Geometry: final body of the model. Coordinates: model frame, mm. Face numbers are marked on the shaded views. A direction names the side the tool comes from. Give positions to 0.01 mm unless a question says otherwise; leave off trailing zeros. Write each loop counter-clockwise with the first axis right and the second up, starting at its lowest first coordinate (ties: lowest second). Pieces come first, ordered by that corner, then holes.
Q1. Line query: line 1 (Z direction, x = -27, y = -7); line 2 (Y direction, x = 0, z = 3.65); line 3 (X direction, y = -13, z = -27.5). Output: solid intervals per line, ascending.
Q2. Pin query (flat end, axial travel): pin 1 Ø1 at (x, y) = (-5.5, 3.5) entering from -Z; pin 2 Ø3 at (y, z) = (19.5, -55.5) entering from +X; pin 3 Ø15 at (x, y) = (-15, 6) entering from +Z. Return the tip coordinate at first contact, or that it passes through.
Q3. Section A-A (z = -64). Return the cut outline in (x, y), plus the area to 3 significant figures.
Q4. Section D-D (x = -24). Return the cut outline in (y, z).
Q5. Section B-B (y = 13.5). Return the cut outline in (x, z).
Q6. Reachability of the marked faces 1 and 2 from +Z, -Z, +X, -X, +Y, -Y: full face, straight path, thin tool, end or side. Return the list, or none.
Q7. Section C-C (y = 0). Return the cut outline in (x, z).
Q8. Mould query, pull axis Z, two halves, no side actions, for the marked faces 3, 4 and 5. Classes: +Z half, -Z half, draft (parallel to the pull), parting line (faces both ways), or undercut.
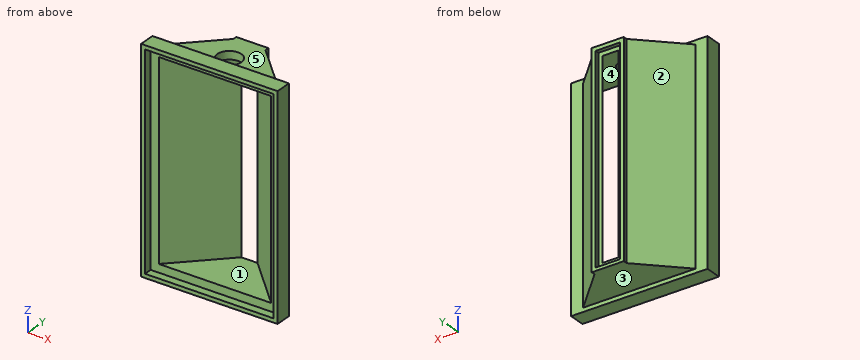
from build123d import *

# Parameters (mm, degrees)
SKETCH2_R            = 7.5
BOSS_EXTRUDE1_DEPTH  = 5
BOSS_EXTRUDE4_DEPTH  = 120
BOSS_EXTRUDE5_DEPTH  = 5
SKETCH7_W            = 85
SKETCH7_H            = 135
SKETCH7_W_2          = 70
SKETCH7_H_2          = 120
BOSS_EXTRUDE6_DEPTH  = 5
SKETCH10_W           = 85
SKETCH10_H           = 135
SKETCH10_W_2         = 80.1
SKETCH10_H_2         = 130.1
BOSS_EXTRUDE9_DEPTH  = 5
SKETCH11_W           = 20
SKETCH11_H           = 130
SKETCH11_W_2         = 15
SKETCH11_H_2         = 125.670447934
BOSS_EXTRUDE10_DEPTH = 2.5


with BuildPart() as part:
    # Sketch2 → Boss-Extrude1 (new body)
    with BuildSketch(Plane.XY):
        Polygon((-10, 17.5), (10, 17.5), (40, -12.5), (-40, -12.5), align=None)
        Circle(SKETCH2_R, mode=Mode.SUBTRACT)
    extrude(amount=BOSS_EXTRUDE1_DEPTH)

    # Sketch5 → Boss-Extrude4 (add)
    with BuildSketch(Plane(origin=(0, 0, 0), x_dir=(-1, 0, 0), z_dir=(0, 0, -1))):
        Polygon((-10, 17.5), (-40, -12.5), (-35, -12.5), (-5, 17.5), align=None)
        Polygon((10, 17.5), (40, -12.5), (35, -12.5), (5, 17.5), align=None)
    extrude(amount=BOSS_EXTRUDE4_DEPTH)

    # Sketch6 → Boss-Extrude5 (add)
    with BuildSketch(Plane(origin=(0, 0, -120), x_dir=(-1, 0, 0), z_dir=(0, 0, -1))):
        Polygon((-40, -12.5), (40, -12.5), (10, 17.5), (-10, 17.5), align=None)
    extrude(amount=BOSS_EXTRUDE5_DEPTH)

    # Sketch7 → Boss-Extrude6 (add)
    with BuildSketch(Plane(origin=(0, -12.5, 0), x_dir=(-1, 0, 0), z_dir=(0, -1, 0))):
        with Locations((0, 60)):
            Rectangle(SKETCH7_W, SKETCH7_H)
        with Locations((0, 60)):
            Rectangle(SKETCH7_W_2, SKETCH7_H_2, mode=Mode.SUBTRACT)
    extrude(amount=-BOSS_EXTRUDE6_DEPTH)

    # Sketch10 → Boss-Extrude9 (add)
    with BuildSketch(Plane(origin=(0, -12.5, 0), x_dir=(-1, 0, 0), z_dir=(0, -1, 0))):
        with Locations((0, 60)):
            Rectangle(SKETCH10_W, SKETCH10_H)
        with Locations((0, 60)):
            Rectangle(SKETCH10_W_2, SKETCH10_H_2, mode=Mode.SUBTRACT)
    extrude(amount=BOSS_EXTRUDE9_DEPTH)

    # Sketch11 → Boss-Extrude10 (add)
    with BuildSketch(Plane(origin=(0, 17.5, 0), x_dir=(1, 0, 0), z_dir=(0, 1, 0))):
        with Locations((0, 60)):
            Rectangle(SKETCH11_W, SKETCH11_H)
        with Locations((0, 60.23315482)):
            Rectangle(SKETCH11_W_2, SKETCH11_H_2, mode=Mode.SUBTRACT)
    extrude(amount=BOSS_EXTRUDE10_DEPTH)


solid = part.part
Computed:
1. line 1: z = -125 to -120, 0 to 5
1. line 2: y = -12.5 to -7.5, 7.5 to 20
1. line 3: x = -42.5 to -40.05, 40.05 to 42.5
2. pin 1: stops at z = -125
2. pin 2: stops at x = 10
2. pin 3: stops at z = 5
3. outline: (-42.5, -17.5) - (-40.05, -17.5) - (-40.05, -12.5) - (-35, -12.5) - (-5, 17.5) - (-7.5, 17.5) - (-7.5, 20) - (-10, 20) - (-10, 17.5) - (-35, -7.5) - (-42.5, -7.5) - close; (5, 17.5) - (35, -12.5) - (40.05, -12.5) - (40.05, -17.5) - (42.5, -17.5) - (42.5, -7.5) - (35, -7.5) - (10, 17.5) - (10, 20) - (7.5, 20) - (7.5, 17.5) - close
3. area: 387 mm2
4. outline: (-17.5, -127.5) - (-7.5, -127.5) - (-7.5, -125) - (3.5, -125) - (3.5, 5) - (-7.5, 5) - (-7.5, 7.5) - (-17.5, 7.5) - (-17.5, 5.05) - (-12.5, 5.05) - (-12.5, 0) - (-1.5, 0) - (-1.5, -120) - (-12.5, -120) - (-12.5, -125.05) - (-17.5, -125.05) - close
5. outline: (-14, -125) - (14, -125) - (14, 5) - (-14, 5) - close; hole (-9, -120) - (9, -120) - (9, 0) - (-9, 0) - close
6. face 1: -Y
6. face 2: +Z, -Z, -X, +Y
7. outline: (-27.5, -125) - (27.5, -125) - (27.5, 5) - (7.5, 5) - (7.5, 0) - (22.5, 0) - (22.5, -120) - (-22.5, -120) - (-22.5, 0) - (-7.5, 0) - (-7.5, 5) - (-27.5, 5) - close
8. face 3: -Z half
8. face 4: undercut
8. face 5: +Z half
